Part model, mm, in its own coordinate system. Face numbers are marked on the shaded views. A direction names the side the tool comes from. Give positions to 0.01 mm unless a question says otherwise; leave off trailing zeros. Order: outer loops, then holes, each group sorted by start corner. A loop starts at its lowest first (then second) coordinate and runs counter-clockwise, first axis right, second up. Notation, with made-up numbers: M -6,-37 L 37,-37 A24 ccw 37,-26 Z; hole C 64,50.25 d8. An arc over 180 degrees is marked long. One line per question, with ' | ' between items.
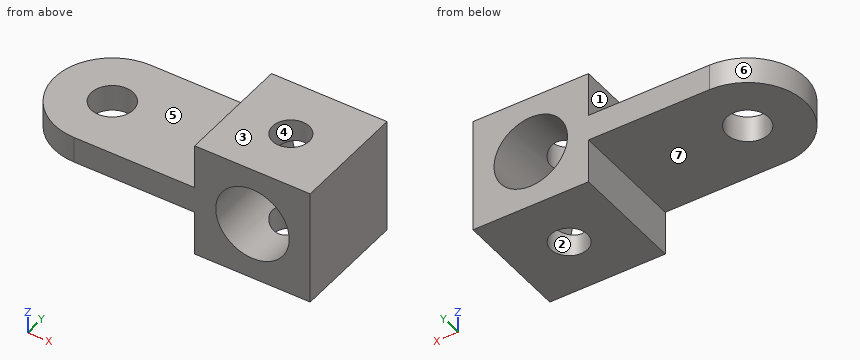
Autodesk Inventor part; units mm, degrees
ref_plane "YZ Plane" through (0, 0, 0) normal (1, 0, 0) x (0, 1, 0)
ref_plane "XZ Plane" through (0, 0, 0) normal (0, 1, 0) x (-1, 0, 0)
ref_plane "XY Plane" through (0, 0, 0) normal (0, 0, 1) x (1, 0, 0)
sketch "Boceto1" plane through (0, 0, 0) normal (0, 1, 0) x (-1, 0, 0)
  line L0 (11, 11) -> (-11, 11)
  line L1 (-11, 11) -> (-11, -11)
  line L2 (-11, -11) -> (11, -11)
  line L3 (11, -11) -> (11, 11)
  line L4 (11, -11) -> (-11, 11) construction
  line L5 (-11, -11) -> (11, 11) construction
  circle A0 centre (0, 0) radius 7 construction
  point P0 (0, 0)
  point P1 (0, 0)
  dimension "d0" = 22
  dimension "d1" = 22
  dimension "d2" = 22
  dimension "d3" = 14
extrude "Extrusión1" add sketch "Boceto1" along normal blind 22
sketch "Boceto2" plane through (0, 0, 0) normal (0, 0, 1) x (1, 0, 0)
  line L0 (0, 0) -> (0, 11) construction
  line L1 (0, 11) -> (-34, 11) construction
  circle A0 centre (-34, 11) radius 4
  arc A1 (-34, 22) -> (-34, 0) centre (-34, 11) ccw
  line L2 (-11, 0) -> (11, 0)
  line L3 (11, 0) -> (11, 22)
  line L4 (-11, 22) -> (11, 22)
  line L5 (-11, 0) -> (-11, 22)
  line L6 (-34, 0) -> (-11, 0)
  line L7 (-34, 22) -> (-11, 22)
  line L8 (-11, 22) -> (-11, 0)
  dimension "d6" = 11
  dimension "d8" = 34
  dimension "d9" = 8
  dimension "d10" = 22
extrude "Extrusión2" add sketch "Boceto2" along normal mid plane 5 contours L7 L5 L6 A1
sketch "Boceto3" plane through (-11, 0, 11) normal (0, 0, 1) x (1, 0, 0)
  line L0 (0, 0) -> (0, 11) construction
  line L1 (0, 0) -> (0, 22)
  line L2 (0, 11) -> (11, 11) construction
  circle A0 centre (11, 11) radius 3.5
  line L3 (0, 0) -> (22, 0)
  point P0 (11, 0)
  point P1 (11, 0)
  dimension "d14" = 7
  dimension "d15" = 11
extrude "Extrusión3" cut sketch "Boceto3" against normal through all
sketch "Boceto4" plane through (0, 22, 0) normal (0, 1, 0) x (1, 0, 0)
  circle A0 centre (0, 0) radius 7
  dimension "d18" = 14
extrude "Extrusión4" cut sketch "Boceto4" against normal through all
properties part number "17_UnionA"
1. Slice it at B-B on x = 0. Give the cut face in (y, z).
Worked out:
outline: M 0,-11 L 7.5,-11 L 7.5,-7 L 0,-7 Z; M 0,7 L 7.5,7 L 7.5,11 L 0,11 Z; M 14.5,-11 L 22,-11 L 22,-7 L 14.5,-7 Z; M 14.5,7 L 22,7 L 22,11 L 14.5,11 Z
2. Slice it at C-C on y = 11. Give the cut face in (x, z).
Worked out:
outline: M -45,-2.5 L -38,-2.5 L -38,2.5 L -45,2.5 Z; M -30,-2.5 L -11,-2.5 L -11,-11 L -3.5,-11 L -3.5,-6.06 A7 cw -3.5,6.06 L -3.5,11 L -11,11 L -11,2.5 L -30,2.5 Z; M 3.5,-11 L 11,-11 L 11,11 L 3.5,11 L 3.5,6.06 A7 cw 3.5,-6.06 Z
3. Slice it at A-A on z = 0. Give the cut face in (x, y), then the cut area to 3 significant figures.
Worked out:
outline: M -34,0 L -7,0 L -7,22 L -34,22 A11 ccw Z; M 7,0 L 11,0 L 11,22 L 7,22 Z; hole C -34,11 d8 | area: 822 mm2
4. Slice it at D-D on z = -8. Give the cut face in (x, y), then the cut area to 3 significant figures.
Worked out:
outline: M -11,0 L 11,0 L 11,22 L -11,22 Z; hole C 0,11 d7 | area: 446 mm2
5. Drop flat-ended pins along their axis: pin 1 (12 mm diameter, centred on x = -23, z = 7, fed in from -Y); pin 2 (1 mm diameter, centred on x = -12.5, y = 17.5, fed in from +Z); pin 3 (9.5 mm diameter, centred on y = 6, z = -7.5, fed in from -X); pin 4 (1 mm diameter, centred on y = 7.5, z = 2.5, fed in from -X). Give the stop position or say it passes through.
Worked out:
pin 1: stops at y = 0 | pin 2: stops at z = 2.5 | pin 3: stops at x = -11 | pin 4: stops at x = -44.58
6. Tool access for the marked faces 5, 6 and 7: list every direction of +Z, -Z, +X, -X, +Y, -Y with a clear straight run to the whole face (end or side of a thin tool).
Worked out:
face 5: +Z, -X, +Y, -Y | face 6: +Z, -Z, -X | face 7: -Z, -X, +Y, -Y
7. Mould opens along X. For the marked faces 1, 2, 3 and 4 say: released by +X, released by -X, zero draft, split by the parting line, or undercut.
Worked out:
face 1: released by -X | face 2: undercut | face 3: zero draft | face 4: undercut
8. Probe L1, parallel to Y at x = -34, z = -0.8; L2, parallel to Y at x = 0, z = 7.75; L3, parallel to X at y = 11, z = 7.6. List the from-to ranges inside material, lowest first. Write a range as from..to.
Worked out:
L1: y = 0..7, 15..22 | L2: y = 0..7.5, 14.5..22 | L3: x = -11..-3.5, 3.5..11
